```python
from build123d import *

# Parameters (mm, degrees)
BOSS_EXTRUDE1_DEPTH     = 20
CIRPATTERN1_COUNT       = 8
SKETCH3_R               = 10
CUT_EXTRUDE1_DEPTH      = 20
CUT_EXTRUDE1_DEPTH_BACK = 7


with BuildPart() as part:
    # Sketch1 → Boss-Extrude1 (new body)
    with BuildSketch(Plane.XY):
        with BuildLine():
            Line((95.877968476, -20.283371538), (78.267729368, -16.557854317))
            ThreePointArc((78.267729368, -16.557854317), (75.247619253, -27.162396743), (70.798070264, -37.250949611))
            Line((70.798070264, -37.250949611), (0, 0))
            Line((0, 0), (76.402194654, 23.721396503))
            Line((76.402194654, 23.721396503), (98, 0))
            ThreePointArc((98, 0), (97.468048382, -10.197036074), (95.877968476, -20.283371538))
        make_face()
    boss_extrude1 = extrude(amount=BOSS_EXTRUDE1_DEPTH)

    # CirPattern1: Boss-Extrude1 ×8 about axis
    cirpattern1_axis = Axis((0, 0, 0), (0, 0, 1))
    for i in range(1, CIRPATTERN1_COUNT):
        add(boss_extrude1.rotate(cirpattern1_axis, i * 360 / CIRPATTERN1_COUNT))

    # Sketch3 → Cut-Extrude1 (cut, two sides)
    with BuildSketch(Plane.XY) as cut_extrude1_sk:
        Circle(SKETCH3_R)
    extrude(amount=CUT_EXTRUDE1_DEPTH, mode=Mode.SUBTRACT)
    extrude(cut_extrude1_sk.sketch, amount=-CUT_EXTRUDE1_DEPTH_BACK, mode=Mode.SUBTRACT)


solid = part.part
```
The listing builds one solid part. Answer for the finished solid, in the listing's coordinates (mm). A direction names the side the tool comes from. Round coordinates to 2 decimals unless told otherwise and drop trailing zeros. Loops run counter-clockwise (first coordinate to the right, second up) from the corner with the lowest first, then second, coordinate; pieces in that order, holes last. Notation, with made-up numbers: (63.25, -36.5) - (70.25, -36.5) arc R31 cw to (70.25, -12.5) - close; hole circle Ø2 at (-7.75, -5.5). An arc over 180 degrees is marked (long way). Return JSON: item names as keys, results as strings. Group by question number.
1. The part is cut by section B-B on x = 7. Determine the outline of the cut face in (y, z), then the cut area to 3 significant figures.
2. Which of the six approach directions +Z, -Z, +X, -X, +Y, -Y give full straight-line access (tool end or side, diameter ignored) to faces 4 (the flat face through (87.05, 12.027, 9.86)), 5 (the flat face through (12.027, -87.05, 9.86)), 6 (the cylindrical face through (-27.02, -75.3, 9.86)), 7 (the cylindrical face through (-97.483, 10.055, 9.86)), 8 (the flat face through (-48.613, 74.701, 9.86))?
3. The mould has two halves that part along Y. Classify faces 1 (the cylindrical face through (-2.17, -9.76, 9.86)), 2 (the flat face through (-13, -15, 0)), 3 (the flat face through (87.196, -18.447, 9.86)): pulls with the +Y half, pulls with the -Y half, needs draft (parallel to the pull), parting line crosses it, or undercut.
4. Consider probe 1 along Y at (x, z) = (9, 3.5); probe 2 along X at (y, z) = (79.5, 15); probe 3 along Y at (x, z) = (-3.5, 3.25). Determine where each line is inside the solid, lowest interval first.
5. Each of these flat-tipped pins is pushed along its axis until it touches: P1, Ø4, axis at y = 10, z = 3.5, coming from the +X side; P2, Ø1.5, axis at x = 54.5, z = 7.5, coming from the -Y side; P3, Ø10, axis at y = 73.5, z = 6.5, coming from the -X side. Where does it stop, or does it pass through?
Resolved:
{
 "1": {"outline": "(-91.63, 0) - (-7.14, 0) - (-7.14, 20) - (-91.63, 20) - close; (7.14, 0) - (97.75, 0) - (97.75, 20) - (7.14, 20) - close", "area": "3,500 mm²"},
 "2": {"face 4": "+Z, -Z, +X", "face 5": "+Z, -Z, -Y", "face 6": "+Z, -Z, -X", "face 7": "+Z, -Z, -X, +Y", "face 8": "+Z, -Z, +Y"},
 "3": {"face 1": "undercut", "face 2": "needs draft", "face 3": "pulls with the -Y half"},
 "4": {"probe 1": "y = -89.81 to -4.36, 4.36 to 97.59", "probe 2": "x = -57.3 to -51.74, -20.32 to 16.82", "probe 3": "y = -97.94 to -9.37, 9.37 to 94.81"},
 "5": {"P1": "stops at x = 90.72", "P2": "stops at y = -81.94", "P3": "stops at x = -69.33"}
}
